Build history of the part. All positions in model axes, mm. Face numbers are marked on the shaded views. A direction names the side the tool comes from. Coordinates: 2 decimals unless noted, no trailing zeros. Loops run counter-clockwise (first coordinate to the right, second up) from the corner with the lowest first, then second, coordinate; pieces in that order, holes last.
Item 1: Flat gauge pins, fed straight in: pin 1 (10 mm diameter, centred on x = 43.5, z = 12, fed in from -Y) (3 decimals); pin 2 (11.5 mm diameter, centred on x = 25.4, y = 8.89, fed in from +Z) (3 decimals). Where does each tip first touch, or does it go through?
Item 2: Cut at B-B (y = 8.89). List the corners of the cut face in (x, z) (3 decimals).
Item 3: Cut at C-C (x = 88). List the corners of the cut face in (y, z) (3 decimals), and give its area (3 significant figures).
Item 4: 3-axis set-ups, long thin cutter, end or side, ignore diameter. For the marked faces 1 and 2: which of +Z, -Z, +X, -X, +Y, -Y reach the whole face in a straight line?
Item 5: Cut at D-D (z = 7). List the corners of the cut face in (x, y) (3 decimals).
Item 6: Cut at A-A (x = 107.95). List the corners of the cut face in (y, z) (3 decimals), and give its area (3 significant figures).
Item 7: Drill centre lines: line 1 along Y through (x, z) = (107.95, 0.9); line 2 along Y through (x, z) = (35, 14) (3 decimals); line 3 along Z through (x, y) = (108, 4.5) (3 decimals). Where is each one in solid material? Low to high.
from build123d import *

# Parameters (mm, degrees)
BOSS_EXTRUDE1_DEPTH = 133.35
SKETCH5_R           = 3.57124
CUT_EXTRUDE1_DEPTH  = 139.103376269


with BuildPart() as part:
    # Sketch1 → Boss-Extrude1 (new body)
    with BuildSketch(Plane(origin=(0, 0, 0), x_dir=(0, 0, -1), z_dir=(1, 0, 0))):
        Polygon((0, 0), (0, 25.4), (-25.4, 25.4), (-25.4, 22.225), (-3.175, 22.225), (-3.175, 0), align=None)
    extrude(amount=BOSS_EXTRUDE1_DEPTH)

    # Cut-Sweep1: read off the stored shape, not the designer's step
    # Cut-Sweep1: loft between two sections, ruled curve by curve
    cut_sweep1_from = [
        Edge.make_bspline([(313.868695545, -367.401209175, 110.125818187), (314.822976006, -368.561544306, 135.48134956), (334.440699372, -352.427576105, 135.48134956), (333.486418911, -351.267240974, 110.125818187), (332.53213845, -350.106905843, 84.770286815), (312.914415084, -366.240874045, 84.770286815), (313.868695545, -367.401209175, 110.125818187)], [0, 0, 0, 0, 0.5, 0.5, 0.5, 1, 1, 1, 1], 3, [1, 0.333333333, 0.333333333, 1, 0.333333333, 0.333333333, 1]),
    ]
    cut_sweep1_to = [
        Edge.make_bspline([(-146.659751189, 323.693531683, -46.998545783), (-145.705470727, 322.533196552, -21.64301441), (-126.087747361, 338.667164754, -21.64301441), (-127.042027823, 339.827499885, -46.998545783), (-127.996308284, 340.987835016, -72.354077155), (-147.61403165, 324.853866814, -72.354077155), (-146.659751189, 323.693531683, -46.998545783)], [0, 0, 0, 0, 0.5, 0.5, 0.5, 1, 1, 1, 1], 3, [1, 0.333333333, 0.333333333, 1, 0.333333333, 0.333333333, 1]),
    ]
    cut_sweep1 = Solid(Shell([*[Face.make_surface_from_curves(cut_sweep1_from[k], cut_sweep1_to[k]) for k in range(1)], Face(Wire(cut_sweep1_from)), Face(Wire(cut_sweep1_to))]))
    add(cut_sweep1, mode=Mode.SUBTRACT)

    # Sketch5 → Cut-Extrude1 (cut, through all)
    with BuildSketch(Plane(origin=(0, 0, 0), x_dir=(-1, 0, 0), z_dir=(0, 0, -1))):
        with Locations((-107.95, 8.89)):
            Circle(SKETCH5_R)
        with Locations((-25.4, 8.89)):
            Circle(SKETCH5_R)
    extrude(amount=-CUT_EXTRUDE1_DEPTH, mode=Mode.SUBTRACT)


solid = part.part
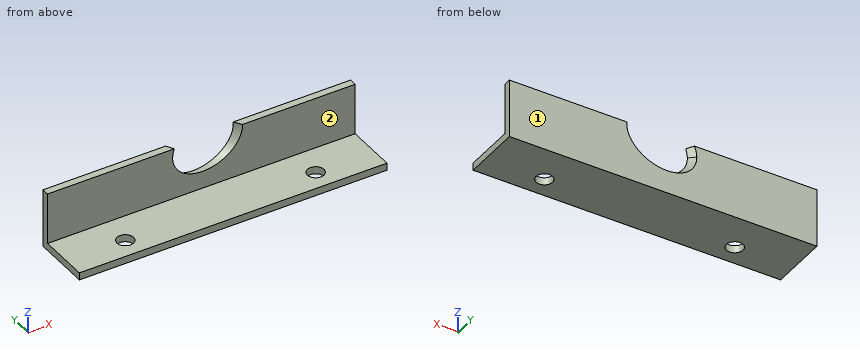
Filled sheet:
1. pin 1: stops at y = 22.225
1. pin 2: stops at z = 3.175
2. outline: (0, 0) - (21.829, 0) - (21.829, 3.175) - (0, 3.175) - close; (28.971, 0) - (104.379, 0) - (104.379, 3.175) - (28.971, 3.175) - close; (111.521, 0) - (133.35, 0) - (133.35, 3.175) - (111.521, 3.175) - close
3. outline: (0, 0) - (25.4, 0) - (25.4, 25.4) - (22.225, 25.4) - (22.225, 3.175) - (0, 3.175) - close
3. area: 151 mm2
4. face 1: +Z, -Z, +X, -X, +Y
4. face 2: +Z, +X, -X, -Y
5. outline: (0, 22.225) - (133.35, 22.225) - (133.35, 25.4) - (0, 25.4) - close
6. outline: (0, 0) - (5.319, 0) - (5.319, 3.175) - (0, 3.175) - close; (12.461, 0) - (25.4, 0) - (25.4, 25.4) - (22.225, 25.4) - (22.225, 3.175) - (12.461, 3.175) - close
6. area: 129 mm2
7. line 1: y = 0 to 5.32, 12.46 to 25.4
7. line 2: y = 22.225 to 25.4
7. line 3: z = 0 to 3.175
